CAD build for the part. Positions are in the model's coordinates, mm. A direction names the side the tool comes from. Round coordinates to 2 decimals unless told otherwise and drop trailing zeros. Loops run counter-clockwise (first coordinate to the right, second up) from the corner with the lowest first, then second, coordinate; pieces in that order, holes last.
Autodesk Inventor part; units mm, degrees
ref_plane "YZ Plane" through (0, 0, 0) normal (1, 0, 0) x (0, 1, 0)
ref_plane "XZ Plane" through (0, 0, 0) normal (0, 1, 0) x (-1, 0, 0)
ref_plane "XY Plane" through (0, 0, 0) normal (0, 0, 1) x (1, 0, 0)
sketch "Sketch1" plane through (0, 0, 0) normal (0, 0, 1) x (1, 0, 0)
  circle A0 centre (0, 0) radius 3.125
  dimension "d0" = 6.25
extrude "Extrusion1" add sketch "Sketch1" along normal blind 20
sketch "Sketch2" plane through (0, 0, 0) normal (0, 0, -1) x (-1, 0, 0)
  circle A0 centre (0, 0) radius 19
  dimension "d3" = 38
extrude "Extrusion2" add sketch "Sketch2" along normal blind 2
sketch "Sketch3" plane through (0, 0, -2) normal (0, 0, -1) x (-1, 0, 0)
  circle A0 centre (0, 0) radius 3.125
  line L0 (27.75, 27.75) -> (-27.75, 27.75)
  line L1 (-27.75, 27.75) -> (-27.75, -27.75)
  line L2 (-27.75, -27.75) -> (27.75, -27.75)
  line L3 (27.75, -27.75) -> (27.75, 27.75)
  point P0 (27.75, 0)
  point P1 (0, 27.75)
  dimension "d6" = 55.5
extrude "Extrusion3" add sketch "Sketch3" along normal blind 5
fillet "Fillet1" radius 2.5 4 edges at (27.75, 27.75, -4.5) (-27.75, 27.75, -4.5) (-27.75, -27.75, -4.5) (27.75, -27.75, -4.5)
sketch "Sketch4" plane through (0, 0, -2) normal (0, 0, 1) x (1, 0, 0)
  arc A0 (25.25, -27.75) -> (27.75, -25.25) centre (25.25, -25.25) ccw
  line L0 (27.75, 25.25) -> (27.75, -25.25)
  arc A1 (27.75, 25.25) -> (25.25, 27.75) centre (25.25, 25.25) ccw
  line L1 (-25.25, 27.75) -> (25.25, 27.75)
  arc A2 (-25.25, 27.75) -> (-27.75, 25.25) centre (-25.25, 25.25) ccw
  line L2 (-27.75, -25.25) -> (-27.75, 25.25)
  arc A3 (-27.75, -25.25) -> (-25.25, -27.75) centre (-25.25, -25.25) ccw
  line L3 (25.25, -27.75) -> (-25.25, -27.75)
  circle A4 centre (0, 0) radius 19
  line L4 (-22.5, 22.5) -> (22.5, 22.5) construction
  line L5 (22.5, 22.5) -> (22.5, -22.5) construction
  line L6 (22.5, -22.5) -> (-22.5, -22.5) construction
  line L7 (-22.5, -22.5) -> (-22.5, 22.5) construction
  circle A5 centre (22.5, 22.5) radius 2.75
  circle A6 centre (-22.5, 22.5) radius 2.75
  circle A7 centre (-22.5, -22.5) radius 2.75
  circle A8 centre (22.5, -22.5) radius 2.75
  point P0 (-22.5, 0)
  point P1 (0, 22.5)
  dimension "d10" = 45
  dimension "d11" = 5.5
extrude "Extrusion4" cut sketch "Sketch4" against normal through all contours A5 | A6 | A7 | A8
sketch "Sketch5" plane through (0, 0, -7) normal (0, 0, -1) x (-1, 0, 0)
  circle A0 centre (22.5, -22.5) radius 2.75 construction
  circle A1 centre (-22.5, 22.5) radius 2.75 construction
  circle A2 centre (22.5, 22.5) radius 2.75 construction
  circle A3 centre (-22.5, -22.5) radius 2.75 construction
  arc A4 (-27.75, -25.25) -> (-25.25, -27.75) centre (-25.25, -25.25) ccw construction
  line L0 (-25.25, -27.75) -> (25.25, -27.75) construction
  arc A5 (25.25, -27.75) -> (27.75, -25.25) centre (25.25, -25.25) ccw construction
  line L1 (27.75, -25.25) -> (27.75, 25.25) construction
  arc A6 (27.75, 25.25) -> (25.25, 27.75) centre (25.25, 25.25) ccw construction
  line L2 (25.25, 27.75) -> (-25.25, 27.75) construction
  arc A7 (-25.25, 27.75) -> (-27.75, 25.25) centre (-25.25, 25.25) ccw construction
  line L3 (-27.75, 25.25) -> (-27.75, -25.25) construction
  circle A8 centre (0, 0) radius 3.125 construction
  circle A9 centre (22.5, 22.5) radius 2.75
  arc A10 (20.8606, 27.75) -> (27.75, 20.8606) centre (22.5, 22.5) ccw
  arc A11 (27.75, -20.8606) -> (20.8606, -27.75) centre (22.5, -22.5) ccw
  arc A12 (-20.8606, -27.75) -> (-27.75, -20.8606) centre (-22.5, -22.5) ccw
  arc A13 (-27.75, 20.8606) -> (-20.8606, 27.75) centre (-22.5, 22.5) ccw
  line L4 (27.75, 20.8606) -> (27.75, -20.8606)
  line L5 (20.8606, 27.75) -> (-20.8606, 27.75)
  line L6 (25.25, 27.75) -> (-25.25, 27.75) construction
  line L7 (-27.75, 20.8606) -> (-27.75, -20.8606)
  line L8 (-27.75, 25.25) -> (-27.75, -25.25) construction
  line L9 (-20.8606, -27.75) -> (20.8606, -27.75)
  dimension "d14" = 11
extrude "Extrusion5" add sketch "Sketch5" along normal blind 75 contours A10 L4 A11 L9 A12 L7 A13 L5
fillet "Fillet2" radius 2 8 edges at (20.8606, 27.75, -44.5) (27.75, 20.8606, -44.5) (-20.8606, 27.75, -44.5) (-27.75, 20.8606, -44.5) (20.8606, -27.75, -44.5) (27.75, -20.8606, -44.5) (-20.8606, -27.75, -44.5) (-27.75, -20.8606, -44.5)
properties part number "NEMA23" material "Titanium"
Item 1: Cut at D-D (z = 8.5). List the corners of the cut face in (x, y) (3 decimals).
Verdict:
outline: circle Ø6.25 at (0, 0)
Item 2: Wall check: L1, parallel to Y at x = 22.5, z = -5.3; L2, parallel to Y at x = 0, z = -5.95 (3 decimals); L3, parallel to X at y = 22, z = -4. Give the ranges that are in metal, low to high.
Verdict:
L1: y = -27.75 to -25.25, -19.75 to 19.75, 25.25 to 27.75
L2: y = -27.75 to -3.125, 3.125 to 27.75
L3: x = -27.75 to -25.2, -19.8 to 19.8, 25.2 to 27.75
Item 3: Mould opens along Y. For faces 1 (the cylindrical face through (-25.247, -22.379, -4.465)), 2 (the cylindrical face through (-26.79, -17.45, -45.02)), 3 (the cylindrical face through (26.998, 27.037, -4.535)), 4 (the flat face through (0, 0, -82)) say: released by +Y, released by -Y, zero draft, split by the parting line, or undercut.
Verdict:
face 1: undercut
face 2: released by -Y
face 3: released by +Y
face 4: zero draft
Item 4: 3-axis set-ups, long thin cutter, end or side, ignore diameter. For faces 5 (the cylindrical face through (18.544, 18.679, -43.975)), 6 (the cylindrical face through (17.45, -26.79, -45.02)), 7 (the cylindrical face through (26.838, -17.419, -45.025)), 8 (the cylindrical face through (-17.45, 26.79, -45.02)): which of +Z, -Z, +X, -X, +Y, -Y reach the whole face in a straight line?
Verdict:
face 5: -Z
face 6: -Z, +X
face 7: -Z, -Y
face 8: -Z, -X
Item 5: Cut at B-B (x = 0). List the corners of the cut face in (y, z) (3 decimals).
Verdict:
outline: (-27.75, -82) - (27.75, -82) - (27.75, -2) - (19, -2) - (19, 0) - (3.125, 0) - (3.125, 20) - (-3.125, 20) - (-3.125, 0) - (-19, 0) - (-19, -2) - (-27.75, -2) - close; hole (-3.125, -7) - (3.125, -7) - (3.125, -2) - (-3.125, -2) - close
Item 6: Cut at A-A (y = 22.5). List the corners of the cut face in (x, z), plus the area to 3 significant figures.
Verdict:
outline: (-27.75, -7) - (-25.25, -7) - (-25.25, -2) - (-27.75, -2) - close; (-19.75, -7) - (-17, -7) - (-17, -82) - (17, -82) - (17, -7) - (19.75, -7) - (19.75, -2) - (-19.75, -2) - close; (25.25, -7) - (27.75, -7) - (27.75, -2) - (25.25, -2) - close
area: 2,770 mm2
Item 7: Flat gauge pins, fed straight in: P1, Ø2, axis at x = -16.5, y = 6.5, coming from the +Z side; P2, Ø6, axis at x = 24.5, y = 23, coming from the -Z side; P3, Ø7, axis at x = 22.5, y = 22.5, coming from the +Z side; P4, Ø5, axis at x = -22.5, y = 22.5, coming from the +Z side. Where does each tip first touch, or does it go through?
Verdict:
P1: stops at z = 0
P2: stops at z = -7
P3: stops at z = -2
P4: passes through
